For this review, take the finished solid that the model builds, in its own axes (mm). A direction names the side the tool comes from. Give positions to 0.01 mm unless a question says otherwise; leave off trailing zeros. Loops run counter-clockwise (first coordinate to the right, second up) from the corner with the lowest first, then second, coordinate; pieces in that order, holes last.
```python
from build123d import *

# Parameters (mm, degrees)
BOSS_EXTRUDE1_DEPTH     = 2.5
BOSS_EXTRUDE2_DEPTH     = 3.4
CUT_EXTRUDE1_DEPTH      = 1
CUT_EXTRUDE1_DEPTH_BACK = 10.9
CUT_EXTRUDE2_DEPTH      = 10.810262799
CUT_EXTRUDE2_DEPTH_BACK = 6
SKETCH5_W               = 10
SKETCH5_H               = 1.7
CUT_EXTRUDE3_DEPTH      = 10.810262799
CUT_EXTRUDE3_DEPTH_BACK = 6
SKETCH6_R               = 1
CUT_EXTRUDE4_DEPTH      = 1
CUT_EXTRUDE4_DEPTH_BACK = 10.9
FILLET1_R               = 10
FILLET2_R               = 3


with BuildPart() as part:
    # Sketch1 → Boss-Extrude1 (new body, symmetric)
    with BuildSketch(Plane.XY):
        Polygon((-14.712036777, 6.5), (8.397963223, 6.5), (28.677963223, 0), (-14.712036777, 0), align=None)
    extrude(amount=BOSS_EXTRUDE1_DEPTH, both=True)

    # Sketch2 → Boss-Extrude2 (add)
    with BuildSketch(Plane.XZ):
        with BuildLine():
            Line((-12.212036777, -2.5), (30.682377195, -2.5))
            Line((30.682377195, -2.5), (41.676502177, 8.002543507))
            ThreePointArc((41.676502177, 8.002543507), (41.757330921, 11.537153346), (38.222721082, 11.617982091))
            Line((38.222721082, 11.617982091), (28.677963223, 2.5))
            Line((28.677963223, 2.5), (-12.212036777, 2.5))
            ThreePointArc((-12.212036777, 2.5), (-14.712036777, 0), (-12.212036777, -2.5))
        make_face()
    extrude(amount=BOSS_EXTRUDE2_DEPTH)

    # Sketch3 → Cut-Extrude1 (cut, two sides)
    with BuildSketch(Plane(origin=(0, 6.5, 0), x_dir=(1, 0, 0), z_dir=(0, 1, 0))) as cut_extrude1_sk:
        with BuildLine():
            ThreePointArc((-14.712036777, 0), (-13.97980373, 1.767766953), (-12.212036777, 2.5))
            Line((-12.212036777, 2.5), (-14.712036777, 2.5))
            Line((-14.712036777, 2.5), (-14.712036777, 0))
        make_face()
        with BuildLine():
            ThreePointArc((-12.212036777, -2.5), (-13.97980373, -1.767766953), (-14.712036777, 0))
            Line((-14.712036777, 0), (-14.712036777, -2.5))
            Line((-14.712036777, -2.5), (-12.212036777, -2.5))
        make_face()
    extrude(amount=CUT_EXTRUDE1_DEPTH, mode=Mode.SUBTRACT)
    extrude(cut_extrude1_sk.sketch, amount=-CUT_EXTRUDE1_DEPTH_BACK, mode=Mode.SUBTRACT)

    # Sketch4 → Cut-Extrude2 (cut, two sides)
    with BuildSketch(Plane.XY.offset(2.5)) as cut_extrude2_sk:
        Polygon((-14.712036777, 2.8), (8.310958279, 2.8), (27.654958279, -3.4), (-14.712036777, -3.4), align=None)
    extrude(amount=CUT_EXTRUDE2_DEPTH, mode=Mode.SUBTRACT)
    extrude(cut_extrude2_sk.sketch, amount=-CUT_EXTRUDE2_DEPTH_BACK, mode=Mode.SUBTRACT)

    # Sketch5 → Cut-Extrude3 (cut, two sides)
    with BuildSketch(Plane.XY.offset(2.5)) as cut_extrude3_sk:
        with Locations((-9.712036777, 4.65)):
            Rectangle(SKETCH5_W, SKETCH5_H)
    extrude(amount=CUT_EXTRUDE3_DEPTH, mode=Mode.SUBTRACT)
    extrude(cut_extrude3_sk.sketch, amount=-CUT_EXTRUDE3_DEPTH_BACK, mode=Mode.SUBTRACT)

    # Sketch6 → Cut-Extrude4 (cut, two sides)
    with BuildSketch(Plane(origin=(0, 6.5, 0), x_dir=(1, 0, 0), z_dir=(0, 1, 0))) as cut_extrude4_sk:
        with Locations((-12.212036777, 0)):
            Circle(SKETCH6_R)
        with Locations((39.94961163, -9.810262799)):
            Circle(SKETCH6_R)
    extrude(amount=CUT_EXTRUDE4_DEPTH, mode=Mode.SUBTRACT)
    extrude(cut_extrude4_sk.sketch, amount=-CUT_EXTRUDE4_DEPTH_BACK, mode=Mode.SUBTRACT)

    # Fillet1
    fillet1_edges = [part.edges().sort_by_distance(p)[0] for p in [
        (28.677963223, 0, 0),
        (8.397963223, 6.5, 0),
        (27.654958279, -3.4, 0),
        (8.310958279, 2.8, 0),
    ]]
    fillet(fillet1_edges, radius=FILLET1_R)

    # Fillet2
    fillet2_edges = [part.edges().sort_by_distance(p)[0] for p in [
        (30.682377195, -1.7, -2.5),
        (28.677963223, -1.631211096, 2.5),
    ]]
    fillet(fillet2_edges, radius=FILLET2_R)


solid = part.part
```
Item 1: Take a section at A-A on y = -1. Give the boundary of the cut face in (x, z).
Answer:
outline: (20.17, -2.5) - (29.48, -2.5) arc R3 ccw to (31.55, -1.67) - (41.68, 8) arc R2.5 ccw to (38.22, 11.62) - (29.55, 3.33) arc R3 cw to (27.48, 2.5) - (20.17, 2.5) - close; hole circle Ø2 at (39.95, 9.81)
Item 2: Take a section at B-B on x = -2. Give the boundary of the cut face in (y, z).
Answer:
outline: (2.8, -2.5) - (6.5, -2.5) - (6.5, 2.5) - (2.8, 2.5) - close
Item 3: Tool access review of faces 1 (the cylindrical face through (41.79, -1.68, 11.5)), 2 (the flat face through (36, 0, 5)): name each direction out of +Z, -Z, +X, -X, +Y, -Y from which nothing blocks a thin tool from reaching the whole face with its end or side.
Answer:
face 1: +Y, -Y
face 2: +Z, -Z, +X, +Y
Item 4: The part is to be moulded in two halves that separate along Y. For faces 3 (the flat face through (17.868, -0.263, 0.035)), 4 (the flat face through (-10, 3.8, 0)), 5 (the flat face through (-4.712, 5, 0)), 6 (the cylindrical face through (38.95, -1.68, 9.77)), say which applies: released by +Y, released by -Y, zero draft, split by the parting line, or undercut.
Answer:
face 3: released by -Y
face 4: undercut
face 5: undercut
face 6: zero draft
Item 5: Take a section at C-C on y = 5. Give the boundary of the cut face in (x, z), and give its area (4 significant figures).
Answer:
outline: (-4.71, -2.5) - (13.08, -2.5) - (13.08, 2.5) - (-4.71, 2.5) - close
area: 88.95 mm2
Item 6: For L1, parallel to Y at x = 39.5, z = 11.5; L2, parallel to Z at x = 16, y = 1.5; L3, parallel to X at y = -1.25, z = 9.25, list the stretches that pass through material, from the lowest coordinate up.
Answer:
L1: y = -3.4 to 0
L2: z = -2.5 to 2.5
L3: x = 35.74 to 39.12, 40.78 to 42.39
Item 7: Clearance check with flat-ended pins moving along their axes: pin 1 Ø1.6 at (x, z) = (-12.21, 0) entering from -Y; pin 2 Ø4 at (x, z) = (-8, -1) entering from -Y; pin 3 Ø3 at (x, z) = (12, 2) entering from +Y; pin 4 Ø0.9 at (y, z) = (5, -1) entering from -X. State where each tip first meets the part, or that it passes through.
Answer:
pin 1: passes through
pin 2: stops at y = 2.8
pin 3: stops at y = 5.83
pin 4: stops at x = -4.71
